from build123d import *

# Parameters (mm, degrees)
SKETCH_R        = 2
PAD_DEPTH       = 3
SKETCH001_W     = 136
SKETCH001_H     = 76
PAD001_DEPTH    = 20
SKETCH002_R     = 1.25
POCKET_DEPTH    = 23
SKETCH003_R     = 2.75
SKETCH003_W     = 15
SKETCH003_H     = 8
POCKET001_DEPTH = 5


with BuildPart() as part:
    # Sketch → Pad (new body)
    with BuildSketch(Plane.XY):
        with BuildLine():
            Line((-58, 48), (58, 48))
            ThreePointArc((68, 38), (65.071068, 45.071068), (58, 48))
            Line((68, 38), (68, -38))
            ThreePointArc((58, -48), (65.071068, -45.071068), (68, -38))
            Line((58, -48), (-58, -48))
            ThreePointArc((-68, -38), (-65.071068, -45.071068), (-58, -48))
            Line((-68, -38), (-68, 38))
            ThreePointArc((-58, 48), (-65.071068, 45.071068), (-68, 38))
        make_face()
        with Locations((-51, 43)):
            Circle(SKETCH_R, mode=Mode.SUBTRACT)
        with Locations((51, 43)):
            Circle(SKETCH_R, mode=Mode.SUBTRACT)
        with Locations((-51, -43)):
            Circle(SKETCH_R, mode=Mode.SUBTRACT)
        with Locations((51, -43)):
            Circle(SKETCH_R, mode=Mode.SUBTRACT)
    extrude(amount=PAD_DEPTH)

    # Sketch001 (on Face14 of Pad) → Pad001 (join)
    with BuildSketch(Plane.XY.offset(3)):
        Rectangle(SKETCH001_W, SKETCH001_H)
        Polygon((-60, 36), (60, 36), (60, 30), (66, 30), (66, -30), (60, -30), (60, -36), (-60, -36), (-60, -30), (-66, -30), (-66, 30), (-60, 30), align=None, mode=Mode.SUBTRACT)
    extrude(amount=PAD001_DEPTH)

    # Sketch002 → Pocket (cut)
    with BuildSketch(Plane.XY.offset(23)):
        with Locations((63, -33)):
            Circle(SKETCH002_R)
        with Locations((-63, -33)):
            Circle(SKETCH002_R)
        with Locations((-63, 33)):
            Circle(SKETCH002_R)
        with Locations((63, 33)):
            Circle(SKETCH002_R)
    extrude(amount=-POCKET_DEPTH, mode=Mode.SUBTRACT)

    # Sketch003 (on Face24 of Pocket) → Pocket001 (cut)
    with BuildSketch(Plane.YZ.offset(68)):
        with Locations((-20, 16)):
            Circle(SKETCH003_R)
        with Locations((14.5, 8)):
            Rectangle(SKETCH003_W, SKETCH003_H)
    extrude(amount=-POCKET001_DEPTH, mode=Mode.SUBTRACT)


solid = part.part
Can you work these out from the model? Positions are in its coordinate system, mm. A direction names the side the tool comes from. Coordinates: 2 decimals unless noted, no trailing zeros. Order: outer loops, then holes, each group sorted by start corner. A loop starts at its lowest first (then second) coordinate and runs counter-clockwise, first axis right, second up. Notation, with made-up numbers: M 21,79.5 L 35,79.5 A23 cw 35,110.5 Z; hole C 66.5,28 d2. An arc over 180 degrees is marked long. Answer as CSV lines item,"result".
(1) I'm going to push flat-ended pins straight in: pin 1 (3 mm diameter, centred on x = 11, y = -4.5, fed in from +Z); pin 2 (8 mm diameter, centred on x = 6, z = 13.5, fed in from +Y); pin 3 (10 mm diameter, centred on x = 1.5, z = 13.5, fed in from -Y). Where does each tip first touch, or does it pass through?
Geometry check:
pin 1,"z = 3"
pin 2,"y = 38"
pin 3,"y = -38"
(2) If we mould it in two halves opening along Y, with no side actions, what happens to faces 5 (the flat face through (63, -30, 13)), 6 (the flat face through (-0.3, -36.4, 23)), 7 (the cylindrical face through (65.15, 44.99, 1.48))? For each: released by +Y, released by -Y, zero draft, split by the parting line, or undercut.
Geometry check:
face 5,"undercut"
face 6,"zero draft"
face 7,"released by +Y"
(3) On a 3-axis mill with a long thin cutter (end or side, diameter ignored), from which of +Z, -Z, +X, -X, +Y, -Y can I reach the whole of each face in a straight line? I mean faces 1 (the cylindrical face through (67.014, -22.747, 16.121)), 2 (the flat face through (1, 43, 3)), 3 (the flat face through (60, -33, 13)), 4 (the flat face through (1, -43, 3)). Say none if no direction works.
Geometry check:
face 1,"+X"
face 2,"+Z, +X, -X, +Y"
face 3,"+Z"
face 4,"+Z, +X, -X, -Y"
(4) Suppose I cut it at A-A on z = 16. Please give me the cut outline in (x, y), plus the area to 3 significant figures.
Geometry check:
outline,"M -68,-38 L 68,-38 L 68,-22.75 L 66,-22.75 L 66,-30 L 60,-30 L 60,-36 L -60,-36 L -60,-30 L -66,-30 L -66,30 L -60,30 L -60,36 L 60,36 L 60,30 L 66,30 L 66,-17.25 L 68,-17.25 L 68,38 L -68,38 Z; hole C -63,-33 d2.5; hole C -63,33 d2.5; hole C 63,-33 d2.5; hole C 63,33 d2.5"
area,"945 mm^2"
(5) Suppose I cut it at D-D on z = 7. Please give me the cut outline in (x, y), plus the area to 3 significant figures.
Geometry check:
outline,"M -68,-38 L 68,-38 L 68,7 L 66,7 L 66,-30 L 60,-30 L 60,-36 L -60,-36 L -60,-30 L -66,-30 L -66,30 L -60,30 L -60,36 L 60,36 L 60,30 L 66,30 L 66,22 L 68,22 L 68,38 L -68,38 Z; hole C -63,-33 d2.5; hole C -63,33 d2.5; hole C 63,-33 d2.5; hole C 63,33 d2.5"
area,"926 mm^2"
(6) Suppose I cut it at B-B on x = 51. Please give me the cut outline in (y, z).
Geometry check:
outline,"M -48,0 L -45,0 L -45,3 L -48,3 Z; M -41,0 L 41,0 L 41,3 L 38,3 L 38,23 L 36,23 L 36,3 L -36,3 L -36,23 L -38,23 L -38,3 L -41,3 Z; M 45,0 L 48,0 L 48,3 L 45,3 Z"
(7) Please list where these lines run through material, in increasing order: L1, parallel to Y at x = -63, z = 10.75; L2, parallel to Y at x = -11, z = 19.5; L3, parallel to X at y = 10, z = 15.25.
Geometry check:
L1,"-38 to -34.25, -31.75 to -30, 30 to 31.75, 34.25 to 38"
L2,"-38 to -36, 36 to 38"
L3,"-68 to -66, 66 to 68"
(8) Suppose I cut it at C-C on x = -15.5. Please give me the cut outline in (y, z), plus the area to 3 significant figures.
Geometry check:
outline,"M -48,0 L 48,0 L 48,3 L 38,3 L 38,23 L 36,23 L 36,3 L -36,3 L -36,23 L -38,23 L -38,3 L -48,3 Z"
area,"368 mm^2"
